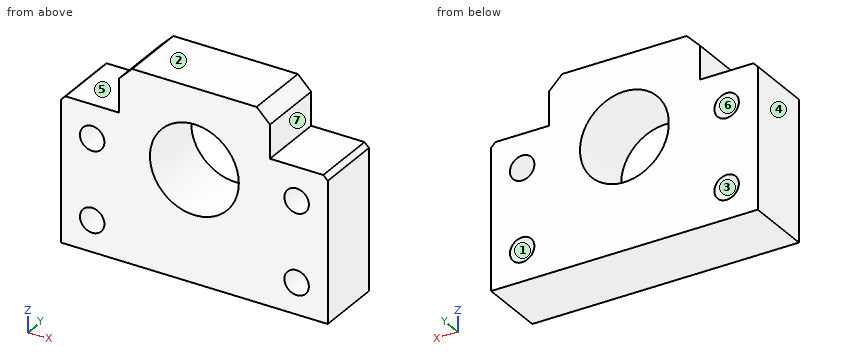
from build123d import *

# Parameters (mm, degrees)
F1_DEPTH = 7.5
F2_R     = 10
F2_R_2   = 2.75
F3_DEPTH = 15
F4_SIZE  = 3
F5_SIZE  = 1


with BuildPart() as f1:
    # F0 (on Front) → F1 (new body, symmetric)
    with BuildSketch(Plane.XZ):
        Polygon((17, 11), (17, 21.5), (-17, 21.5), (-17, 11), (-30, 11), (-30, -21.5), (30, -21.5), (30, 11), align=None)
    extrude(amount=F1_DEPTH, both=True)

    # F2 (on face) → F3 (cut)
    with BuildSketch(Plane.XZ.offset(7.5)):
        with Locations((0, 3.5)):
            Circle(F2_R)
        with Locations((-23, 3.5)):
            Circle(F2_R_2)
        with Locations((23, 3.5)):
            Circle(F2_R_2)
        with Locations((-23, -14.5)):
            Circle(F2_R_2)
        with Locations((23, -14.5)):
            Circle(F2_R_2)
    extrude(amount=-F3_DEPTH, mode=Mode.SUBTRACT)

    # F4
    f4_edges = [f1.edges().sort_by_distance(p)[0] for p in [
        (17, 0, 21.5),
        (-17, 0, 21.5),
    ]]
    chamfer(f4_edges, length=F4_SIZE)

    # F5
    f5_edges = [f1.edges().sort_by_distance(p)[0] for p in [
        (-30, 0, 11),
        (30, 0, 11),
    ]]
    chamfer(f5_edges, length=F5_SIZE)


solid = f1.part
Work out the finished part from the listing and answer in its coordinate system (mm). Face numbers are marked on the shaded views. A direction names the side the tool comes from. Round coordinates to 2 decimals unless told otherwise and drop trailing zeros. Write each loop counter-clockwise with the first axis right and the second up, starting at its lowest first coordinate (ties: lowest second). Pieces come first, ordered by that corner, then holes. Notation, with made-up numbers: (27, 23) - (67, 23) arc R22 ccw to (67, 31) - close; hole circle Ø10 at (34.5, 77). An arc over 180 degrees is marked (long way). Answer in a Markdown table with one row per item. Add a question column.
1. A cutting plane is placed at A-A, the plane z = 3.5. Determine the outline of the cut face in (x, y).
2. Given pin 1 (8 mm diameter, centred on y = -0.5, z = 14.5, fed in from +X); pin 2 (6.5 mm diameter, centred on x = 23, z = 3.5, fed in from +Y); pin 3 (2 mm diameter, centred on y = 0.5, z = 14.5, fed in from -X); pin 4 (6 mm diameter, centred on x = -23.5, y = 3, fed in from +Z), each flat-ended and moving along its own axis, determine where each tip first touches the part or whether it passes through.
3. A cutting plane is placed at B-B, the plane x = -23. Determine the outline of the cut face in (y, z), and give its area (4 significant figures).
4. Find the intervals of material crossed by line 1 along Z through (x, y) = (-23, 1.5); line 2 along Z through (x, y) = (20.5, -6); line 3 along X through (y, z) = (-3.5, -14), in increasing order. Write a range as from..to.
5. A cutting plane is placed at D-D, the plane y = 4. Determine the outline of the cut face in (x, z), and give its area (3 significant figures).
6. A cutting plane is placed at C-C, the plane x = 0. Determine the outline of the cut face in (y, z).
7. For the marked faces 5, 6 and 7, determine the directions among +Z, -Z, +X, -X, +Y, -Y from which every point of the face is accessible in a straight line to the end or side of a thin tool.
8. The mould has two halves that part along Z. Classify the marked faces 1, 2, 3 and 4: +Z half, -Z half, draft (parallel to the pull), parting line (faces both ways), or undercut.
Worked out:
| question | item | result |
|---|---|---|
| 1 | outline | (-30, -7.5) - (-25.75, -7.5) - (-25.75, 7.5) - (-30, 7.5) - close; (-20.25, -7.5) - (-10, -7.5) - (-10, 7.5) - (-20.25, 7.5) - close; (10, -7.5) - (20.25, -7.5) - (20.25, 7.5) - (10, 7.5) - close; (25.75, -7.5) - (30, -7.5) - (30, 7.5) - (25.75, 7.5) - close |
| 2 | pin 1 | x = 29.5 |
| 2 | pin 2 | y = 7.5 |
| 2 | pin 3 | x = -17 |
| 2 | pin 4 | z = 11 |
| 3 | outline | (-7.5, -21.5) - (7.5, -21.5) - (7.5, -17.25) - (-7.5, -17.25) - close; (-7.5, -11.75) - (7.5, -11.75) - (7.5, 0.75) - (-7.5, 0.75) - close; (-7.5, 6.25) - (7.5, 6.25) - (7.5, 11) - (-7.5, 11) - close |
| 3 | area | 322.5 mm^2 |
| 4 | line 1 | -21.5..-17.25, -11.75..0.75, 6.25..11 |
| 4 | line 2 | -21.5..-15.65, -13.35..2.35, 4.65..11 |
| 4 | line 3 | -30..-25.7, -20.3..20.3, 25.7..30 |
| 5 | outline | (-30, -21.5) - (30, -21.5) - (30, 10) - (29, 11) - (17, 11) - (17, 18.5) - (14, 21.5) - (-14, 21.5) - (-17, 18.5) - (-17, 11) - (-29, 11) - (-30, 10) - close; hole circle Ø5.5 at (-23, -14.5); hole circle Ø5.5 at (-23, 3.5); hole circle Ø20 at (0, 3.5); hole circle Ø5.5 at (23, -14.5); hole circle Ø5.5 at (23, 3.5) |
| 5 | area | 1,890 mm^2 |
| 6 | outline | (-7.5, -21.5) - (7.5, -21.5) - (7.5, -6.5) - (-7.5, -6.5) - close; (-7.5, 13.5) - (7.5, 13.5) - (7.5, 21.5) - (-7.5, 21.5) - close |
| 7 | face 5 | +Z, -X, +Y, -Y |
| 7 | face 6 | +Y, -Y |
| 7 | face 7 | +Z, +X, +Y, -Y |
| 8 | face 1 | undercut |
| 8 | face 2 | +Z half |
| 8 | face 3 | undercut |
| 8 | face 4 | draft |
